Can you work these out from the model? Positions are in its coordinate system, mm. Face numbers are marked on the shaded views. A direction names the side the tool comes from. Give positions to 0.01 mm unless a question says otherwise; leave off trailing zeros. Loops run counter-clockwise (first coordinate to the right, second up) from the corner with the lowest first, then second, coordinate; pieces in that order, holes last. Notation, with made-up numbers: (9, -34) - (48, -34) arc R29 cw to (48, 3) - close; hole circle Ø10 at (8, -37). An arc over 180 degrees is marked (long way). Answer as a JSON object with one key per item and string values.
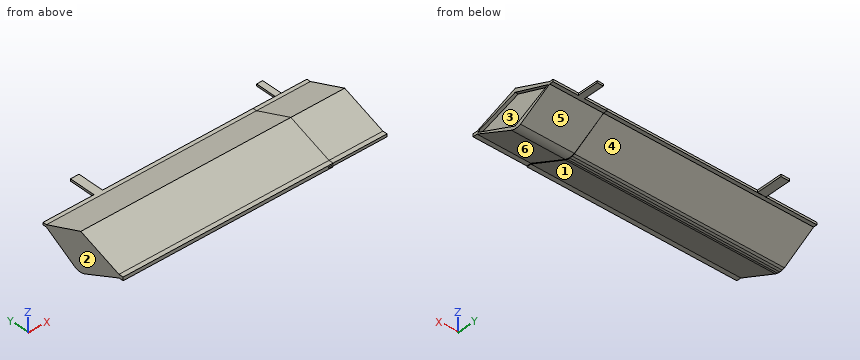
```python
from build123d import *
from build123d.topology import SkipClean

# Parameters (mm, degrees)
SKETCH4_W           = 62.83623107
SKETCH4_H           = 84.722256574
BOSS_EXTRUDE2_DEPTH = 50
CUT_EXTRUDE2_DEPTH  = 80
CUT_EXTRUDE3_DEPTH  = 80
CUT_EXTRUDE5_DEPTH  = 80
CUT_EXTRUDE6_DEPTH  = 3
CUT_EXTRUDE8_DEPTH  = 80
CUT_EXTRUDE9_DEPTH  = 80
SKETCH11_W          = 5.870888161
SKETCH11_H          = 1.865764547
BOSS_EXTRUDE3_DEPTH = 20
SCALE1_SCALE        = 0.5
SCALE2_SCALE        = 0.4
SCALE3_SCALE        = 0.5
SCALE5_SCALE        = 4
BOSS_EXTRUDE5_DEPTH = 80
SKETCH15_W          = 3.250018584
SKETCH15_H          = 0.826724594
BOSS_EXTRUDE6_DEPTH = 10


with BuildPart() as part:
    # Sketch4 → Boss-Extrude2 (new body)
    with BuildSketch(Plane.XY):
        Rectangle(SKETCH4_W, SKETCH4_H)
    extrude(amount=BOSS_EXTRUDE2_DEPTH)

    # Sketch5 → Cut-Extrude2 (cut)
    with BuildSketch(Plane(origin=(31.418115535, 0, 0), x_dir=(0, 0, -1), z_dir=(1, 0, 0))):
        Polygon((-31.846034257, 38.728174008), (-31.846034257, 42.361128287), (-50, 42.361128287), (-50, -42.361128287), (-30.898434646, -42.361128287), (-30.898434646, -37.982426726), (-46.322270236, 2.38891709), align=None)
    extrude(amount=-CUT_EXTRUDE2_DEPTH, mode=Mode.SUBTRACT)

    # Sketch6 → Cut-Extrude3 (cut)
    with BuildSketch(Plane(origin=(31.418115535, 0, 0), x_dir=(0, 0, -1), z_dir=(1, 0, 0))):
        Polygon((-29.655383969, 42.361128287), (-29.655383969, 38.722554473), (-8.776416022, 3.750158878), (-28.328453067, -38.117745), (-28.328453067, -42.361128287), (-27.677514405, -46.625913761), (16.839811583, -52.045359618), (10.267667228, 27.190343951), (3.73953172, 54.484047391), align=None)
    extrude(amount=-CUT_EXTRUDE3_DEPTH, mode=Mode.SUBTRACT)

    # Sketch7 → Cut-Extrude5 (cut)
    with BuildSketch(Plane.ZY.offset(31.418115535)):
        with BuildLine():
            ThreePointArc((13.228873585, 11.208051798), (10.417703783, 4.563945687), (11.71087014, -2.533556863))
            ThreePointArc((11.71087014, -2.533556863), (0.747619784, 5.632177302), (13.228873585, 11.208051798))
        make_face()
    extrude(amount=-CUT_EXTRUDE5_DEPTH, mode=Mode.SUBTRACT)

    # Sketch8 → Cut-Extrude6 (cut)
    with BuildSketch(Plane(origin=(31.418115535, 0, 0), x_dir=(0, 0, -1), z_dir=(1, 0, 0))):
        Polygon((-30.111598921, 36.817435747), (-42.735074125, 2.19595341), (-30.111598921, -36.694083179), (-29.289064541, -37.07820135), (-12.845557678, 2.19595341), align=None)
    extrude(amount=-CUT_EXTRUDE6_DEPTH, mode=Mode.SUBTRACT)

    # Sketch9 → Cut-Extrude8 (cut)
    with BuildSketch(Plane(origin=(0, 0, 29.655383969), x_dir=(-1, 0, 0), z_dir=(0, 0, -1))):
        Polygon((19.869908303, 42.361128287), (19.869908303, 38.722554473), (19.869908303, 5.586987563), (19.869908303, -4.186945454), (19.869908303, -38.208459621), (19.869908303, -42.059759196), (19.869908303, -47.026854784), (41.256673117, -49.585938288), (42.081255469, -21.197702537), (42.081255469, 12.428184914), (37.482224788, 37.513066745), (31.418115535, 49.4837873), align=None)
    extrude(amount=-CUT_EXTRUDE8_DEPTH, mode=Mode.SUBTRACT)

    # Sketch10 → Cut-Extrude9 (cut)
    with BuildSketch(Plane(origin=(0, -2.877407212, 4.819674209), x_dir=(-1, 0, 0), z_dir=(0, 0.5126085745439567, -0.8586224136976701))):
        Polygon((19.869908303, 48.44965729), (25.693686727, -39.803296282), (32.448126733, -43.444815965), (49.802642339, -43.444815965), (32.448126733, 57.840856492), align=None)
    extrude(amount=-CUT_EXTRUDE9_DEPTH, mode=Mode.SUBTRACT)

    # Sketch11 → Boss-Extrude3 (add)
    with BuildSketch(Plane(origin=(0, 42.361128287, 0), x_dir=(1, 0, 0), z_dir=(0, 1, 0))):
        with Locations((4.437413085, -30.588266243)):
            Rectangle(SKETCH11_W, SKETCH11_H)
    extrude(amount=BOSS_EXTRUDE3_DEPTH)


with BuildPart() as part_1:
    # Scale1: scaled about (4.044501914, 0.935318094, 28.406526913)
    add(part.part.scale(SCALE1_SCALE).moved(Location((2.022250957, 0.467659047, 14.203263457))))


with BuildPart() as part_2:
    # Scale2: scaled about (4.044501914, 0.935318094, 28.406526913)
    add(part_1.part.scale(SCALE2_SCALE).moved(Location((2.426701148, 0.561190856, 17.043916148))))


with BuildPart() as part_3:
    # Scale3: scaled about (4.044501914, 0.935318094, 28.406526913)
    add(part_2.part.scale(SCALE3_SCALE).moved(Location((2.022250957, 0.467659047, 14.203263457))))


with BuildPart() as part_4:
    # Scale5: scaled about (4.044501914, 0.935318094, 28.406526913)
    add(part_3.part.scale(SCALE5_SCALE).moved(Location((-12.133505742, -2.805954282, -85.219580739))))


with BuildPart() as boss_extrude5_tool:
    # Sketch14 → Boss-Extrude5 (new body)
    with SkipClean():  # the faces are left unmerged after this step: merging them gives an invalid solid
        with BuildSketch(Plane.ZY.offset(5.521262115)):
            Polygon((28.906071344, 17.505641119), (29.782331459, 17.505641119), (29.782331459, 16.052459408), (35.572825851, 1.51675664), (29.403291615, -14.631780886), (29.403291615, -16.38326151), (28.087210799, -16.38326151), (28.1159044, -14.686132768), (21.408340925, -0.141125859), (21.121993698, 0.799090379), (21.024804823, 1.784179002), (21.121993698, 2.789147348), (21.41419066, 3.732235959), (28.906071344, 16.050211594), align=None)
        extrude(amount=BOSS_EXTRUDE5_DEPTH)


with BuildPart() as part_5:
    with SkipClean():  # the faces are left unmerged after this step: merging them gives an invalid solid
        add(part_4.part)


with BuildPart() as part_6:
    # Boss-Extrude5: joined with boss_extrude5_tool
    with SkipClean():  # the faces are left unmerged after this step: merging them gives an invalid solid
        add(part_5.part.fuse(boss_extrude5_tool.part, tol=0.00001))

    # Sketch15 → Boss-Extrude6 (add)
    with SkipClean():  # the faces are left unmerged after this step: merging them gives an invalid solid
        with BuildSketch(Plane(origin=(0, 17.505641119, 0), x_dir=(1, 0, 0), z_dir=(0, 1, 0))):
            with Locations((-64.439728037, -29.368969162)):
                Rectangle(SKETCH15_W, SKETCH15_H)
        extrude(amount=BOSS_EXTRUDE6_DEPTH)


solid = part_6.part
```
1) I need wall thicknesses on L1, parallel to X at y = -12, z = 29.25; L2, parallel to Z at x = -23, y = 17; L3, parallel to Z at x = -43.5, y = 9.5. Which ranges of each line are inside material? Lowest first, please.
Check sheet entries:
{"L1": "-85.52 to 13.79", "L2": "28.91 to 29.78", "L3": "24.92 to 32.39"}
2) I'm going to push flat-ended pins straight in: P1, Ø0.7, axis at y = 21, z = 29.5, coming from the -X side; P2, Ø0.9, axis at y = 24.5, z = 29.5, coming from the +X side; P3, Ø12.5, axis at x = -47.5, y = 20.5, coming from the +Z side. Where does each tip first touch, or does it pass through?
Check sheet entries:
{"P1": "x = -66.06", "P2": "x = 5.38", "P3": "z = 30.5"}
3) If we mould it in two halves opening along Z, with no side actions, what happens to the marked faces 1, 2 and 3? For each: released by +Z, released by -Z, zero draft, split by the parting line, or undercut.
Check sheet entries:
{"face 1": "released by -Z", "face 2": "zero draft", "face 3": "undercut"}
4) Imagine slicing it at B-B on x = 2. Write out the boundary of the cut face in (y, z), and give its area (3 significant figures).
Check sheet entries:
{"outline": "(-16.38, 28.38) - (-14.69, 28.38) - (-0.15, 21.59) arc R5.04 ccw to (3.73, 21.55) - (16.05, 28.91) - (17.51, 28.91) - (17.51, 29.78) - (16.05, 29.78) - (1.52, 35.57) - (-14.63, 29.4) - (-16.38, 29.4) - close", "area": "248 mm2"}
5) Which directions (+Z, -Z, +X, -X, +Y, -Y) give clear straight access to the entire face, cutting with the end or side of a thin tool? Please do the marked faces 4, 5 and 6.
Check sheet entries:
{"face 4": "-Z, +X, -X, +Y", "face 5": "-Z, +X, +Y", "face 6": "-Z, +X, -Y"}
6) Imagine slicing it at A-A on y = 22. Write out the boundary of the cut face in (x, z).
Check sheet entries:
{"outline": "(-66.06, 28.96) - (-62.81, 28.96) - (-62.81, 29.78) - (-66.06, 29.78) - close; (3.03, 28.91) - (5.38, 28.91) - (5.38, 29.65) - (3.03, 29.65) - close"}
7) Imagine slicing it at D-D on y = 7. Write out the boundary of the cut face in (x, z).
Check sheet entries:
{"outline": "(-85.52, 23.4) - (-5.52, 23.4) - (-5.52, 23.5) - (14.99, 23.5) - (14.99, 24.96) - (13.79, 24.96) - (13.79, 32.11) - (14.99, 32.11) - (14.99, 33.39) - (-85.52, 33.39) - close"}
8) Imagine slicing it at C-C on z = 25.5. Write out the boundary of the cut face in (x, y), and give its area (3 significant figures).
Check sheet entries:
{"outline": "(-85.52, -9.01) - (-5.52, -9.01) - (-5.52, -8.53) - (14.99, -8.53) - (14.99, -6.48) - (13.79, -6.48) - (13.79, 8.09) - (14.99, 8.09) - (14.99, 10.35) - (-5.52, 10.35) - (-5.52, 10.45) - (-85.52, 10.45) - close", "area": "1,930 mm2"}
